For this review, take the finished solid that the model builds, in its own axes (mm). Give positions to 0.01 mm unless a question says otherwise; leave off trailing zeros. Write each loop counter-clockwise with the first axis right and the second up, starting at its lowest first coordinate (ties: lowest second). Pieces come first, ordered by that corner, then holes. Notation, with made-up numbers: M 84.25,-2.75 L 119.25,-2.75 A15 cw 119.25,26.25 Z; hole C 77,69.5 d2. An arc over 180 degrees is marked long. Answer as a JSON object with one key per item and string values. Group by question number.
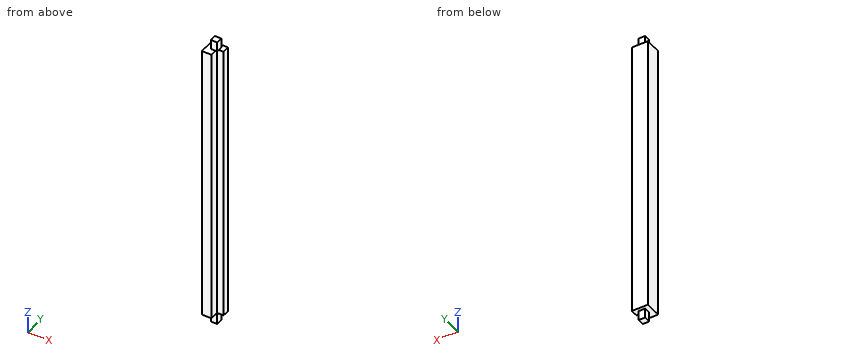
```python
from build123d import *

# Parameters (mm, degrees)
SKETCH2_W           = 5
SKETCH2_H           = 88
BOSS_EXTRUDE1_DEPTH = 5
SKETCH6_W           = 2
SKETCH6_H           = 2
BOSS_EXTRUDE4_DEPTH = 3
SKETCH4_W           = 2
SKETCH4_H           = 2
BOSS_EXTRUDE3_DEPTH = 3
SKETCH5_W           = 2
SKETCH5_H           = 88
CUT_EXTRUDE2_DEPTH  = 2.762


with BuildPart() as part:
    # Sketch2 → Boss-Extrude1 (new body)
    with BuildSketch(Plane(origin=(0, 0, 0), x_dir=(1, 0, 0), z_dir=(0, 1, 0))):
        with Locations((-36.444928995, -11.927663992)):
            Rectangle(SKETCH2_W, SKETCH2_H)
    extrude(amount=BOSS_EXTRUDE1_DEPTH)

    # Sketch6 → Boss-Extrude4 (add)
    with BuildSketch(Plane.XY.offset(55.927663992)):
        with Locations((-36.444928995, 3)):
            Rectangle(SKETCH6_W, SKETCH6_H)
    extrude(amount=BOSS_EXTRUDE4_DEPTH)

    # Sketch4 → Boss-Extrude3 (add)
    with BuildSketch(Plane(origin=(0, 0, -32.072336008), x_dir=(-1, 0, 0), z_dir=(0, 0, -1))):
        with Locations((36.444928995, 3)):
            Rectangle(SKETCH4_W, SKETCH4_H)
    extrude(amount=BOSS_EXTRUDE3_DEPTH)

    # Sketch5 → Cut-Extrude2 (cut)
    with BuildSketch(Plane.XZ):
        with Locations((-34.944928995, 11.927663992)):
            Rectangle(SKETCH5_W, SKETCH5_H)
    extrude(amount=-CUT_EXTRUDE2_DEPTH, mode=Mode.SUBTRACT)


solid = part.part
```
Item 1: Insertion check: P1, Ø1, axis at y = 3, z = 57.5, coming from the -X side; P2, Ø2, axis at y = 1.5, z = 17.5, coming from the +X side; P3, Ø1, axis at y = 2.5, z = 58, coming from the +X side. Each pin has a flat end and moves straight along its axis. Give the tip position at first contact, or say it passes through.
Item 2: Consider section A-A (z = -14). Give the boundary of the cut face in (x, y).
Item 3: To check wall thickness, follow probe 1 along Y at (x, z) = (-35.3, 42.5); probe 2 along X at (y, z) = (2.4, -28); probe 3 along Z at (x, y) = (-36, 1.65). State the ranges of each line that lie inside material, in increasing order.
Item 4: Consider section B-B (y = 0.75). Give the boundary of the cut face in (x, z).
Result set:
{
 "1": {"P1": "stops at x = -37.44", "P2": "stops at x = -35.94", "P3": "stops at x = -35.44"},
 "2": {"outline": "M -38.94,0 L -35.94,0 L -35.94,2.76 L -33.94,2.76 L -33.94,5 L -38.94,5 Z"},
 "3": {"probe 1": "y = 2.76 to 5", "probe 2": "x = -38.94 to -35.94", "probe 3": "z = -32.07 to 55.93"},
 "4": {"outline": "M -38.94,-32.07 L -35.94,-32.07 L -35.94,55.93 L -38.94,55.93 Z"}
}
